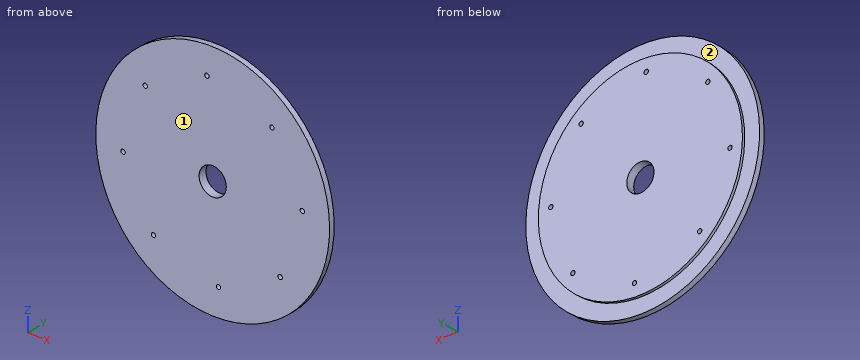
from build123d import *

# Parameters (mm, degrees)
SKETCH_1_R               = 43
EXTRUDE_1_DEPTH          = 1
SKETCH_2_R               = 37.5
EXTRUDE_2_DEPTH          = 1
SKETCH_3_R               = 5
CUT_EXTRUDE_1_DEPTH      = 50
SKETCH_4_R               = 43
SKETCH_4_R_2             = 5
EXTRUDE_3_DEPTH          = 1
SKETCH_5_OUTSIDE_W       = 112.332
SKETCH_5_OUTSIDE_H       = 112.332
SKETCH_5_OUTSIDE_R       = 42.95
CUT_EXTRUDE_2_DEPTH      = 500
SKETCH_6_R               = 0.8
CUT_EXTRUDE_3_DEPTH      = 500
PATTERN_CIRCULAR_1_COUNT = 8


with BuildPart() as part:
    # 草图1 → 凸台-拉伸1 (new body)
    with BuildSketch(Plane(origin=(0, 0, 0), x_dir=(1, 0, 0), z_dir=(0, 1, 0))):
        with Locations(Location((0, 0, 0), (0, 0, 270))):
            Circle(SKETCH_1_R)
    extrude(amount=EXTRUDE_1_DEPTH)

    # 草图2 → 凸台-拉伸2 (add)
    with BuildSketch(Plane(origin=(0, 1, 0), x_dir=(1, 0, 0), z_dir=(0, 1, 0))):
        with Locations(Location((0, 0, 0), (0, 0, 270))):
            Circle(SKETCH_2_R)
    extrude(amount=EXTRUDE_2_DEPTH)

    # 草图3 → 切除-拉伸1 (cut)
    with BuildSketch(Plane(origin=(0, 2, 0), x_dir=(1, 0, 0), z_dir=(0, 1, 0))):
        with Locations(Location((0, 0, 0), (0, 0, 270))):
            Circle(SKETCH_3_R)
    extrude(amount=-CUT_EXTRUDE_1_DEPTH, mode=Mode.SUBTRACT)

    # 草图4 → 凸台-拉伸3 (add)
    with BuildSketch(Plane.XZ):
        with Locations(Location((0, 0, 0), (0, 0, 270))):
            Circle(SKETCH_4_R)
        with Locations(Location((0, 0, 0), (0, 0, 90))):
            Circle(SKETCH_4_R_2, mode=Mode.SUBTRACT)
    extrude(amount=EXTRUDE_3_DEPTH)

    # 草图5 outside → 切除-拉伸2 (cut)
    with BuildSketch(Plane.XZ.offset(1)):
        Rectangle(SKETCH_5_OUTSIDE_W, SKETCH_5_OUTSIDE_H)
        with Locations(Location((0, 0, 0), (0, 0, 270))):
            Circle(SKETCH_5_OUTSIDE_R, mode=Mode.SUBTRACT)
    extrude(amount=-CUT_EXTRUDE_2_DEPTH, mode=Mode.SUBTRACT)

    # 草图6 → 切除-拉伸3 (cut)
    with BuildSketch(Plane.XZ.offset(1)):
        with Locations(Location((24.794413226, -21.776984933, 0), (0, 0, 270))):
            Circle(SKETCH_6_R)
    cut_extrude_3 = extrude(amount=-CUT_EXTRUDE_3_DEPTH, mode=Mode.SUBTRACT)

    # 阵列(圆周)1: 切除-拉伸3 ×8 about axis
    pattern_circular_1_axis = Axis((0, 0, 0), (0, 1, 0))
    for i in range(1, PATTERN_CIRCULAR_1_COUNT):
        add(cut_extrude_3.rotate(pattern_circular_1_axis, i * 360 / PATTERN_CIRCULAR_1_COUNT), mode=Mode.SUBTRACT)


solid = part.part
Geometry check sheet. Reference: the model listing, model coordinates, mm. Face numbers are marked on the shaded views. A direction names the side the tool comes from. Round coordinates to 2 decimals unless told otherwise and drop trailing zeros. Write each loop counter-clockwise with the first axis right and the second up, starting at its lowest first coordinate (ties: lowest second). Pieces come first, ordered by that corner, then holes. Notation, with made-up numbers: (57, 85) - (75, 85) arc R21 cw to (75, 99) - close; hole circle Ø2 at (58.25, 2). An arc over 180 degrees is marked (long way). One line per item, written item: value.
1. Set-up check for the marked faces 1 and 2: record each of +Z, -Z, +X, -X, +Y, -Y from which the full face is reachable in a straight line by a thin tool's end or side.
The answers:
face 1: +Z, -Z, +X, -X, -Y
face 2: +Y
2. Cross-section at D-D on x = 28. Record the boundary of the cut face in (y, z), and give its area (3 significant figures).
The answers:
outline: (-1, -32.57) - (1, -32.57) - (1, -24.94) - (2, -24.94) - (2, 24.94) - (1, 24.94) - (1, 32.57) - (-1, 32.57) - close
area: 180 mm^2
3. Cross-section at C-C on y = 0.35. Give the number of separate pieces and of enclosed holes in the cut face, and give its area (3 significant figures).
The answers:
separate pieces: 1
enclosed holes: 9
area: 5,700 mm^2
4. Cross-section at B-B on x = 0. Record the boundary of the cut face in (y, z), and give its area (3 significant figures).
The answers:
outline: (-1, -42.95) - (1, -42.95) - (1, -37.5) - (2, -37.5) - (2, -5) - (-1, -5) - close; (-1, 5) - (2, 5) - (2, 37.5) - (1, 37.5) - (1, 42.95) - (-1, 42.95) - close
area: 217 mm^2
5. Depth check by flat-ended pin: pin 1 Ø1.4 at (x, z) = (-32.93, -2.13) entering from +Y. Enter the tip coordinate at first touch or a pass-through.
The answers:
pin 1: passes through
6. Cross-section at A-A on z = 0. Record the boundary of the cut face in (x, y).
The answers:
outline: (-42.95, -1) - (-5, -1) - (-5, 2) - (-37.5, 2) - (-37.5, 1) - (-42.95, 1) - close; (5, -1) - (42.95, -1) - (42.95, 1) - (37.5, 1) - (37.5, 2) - (5, 2) - close
7. Scan lines: L1, parallel to Y at x = -25, z = -34; L2, parallel to Z at x = 24.5, y = 0.5; L3, parallel to X at y = -0.6, z = 34. Record each from-to range of solid material in increasing order.
The answers:
L1: y = -1 to 1
L2: z = -35.28 to -22.52, -21.03 to 35.28
L3: x = -26.24 to 26.24
